Part model, mm, in its own coordinate system. A direction names the side the tool comes from. Give positions to 0.01 mm unless a question says otherwise; leave off trailing zeros.
```python
from build123d import *

# Parameters (mm, degrees)
CROQUIS1_R              = 13.5
SALIENTE_EXTRUIR1_DEPTH = 17
CORTAR_EXTRUIR5_START   = -26
CORTAR_EXTRUIR5_DEPTH   = 26
CROQUIS8_R              = 10
SALIENTE_EXTRUIR2_DEPTH = 5
CROQUIS9_R              = 4.5
CORTAR_EXTRUIR6_DEPTH   = 45
CROQUIS10_R             = 6
CORTAR_EXTRUIR8_DEPTH   = 4
CROQUIS12_R             = 15
SALIENTE_EXTRUIR4_DEPTH = 2.5
CORTAR_EXTRUIR9_START   = -25
CROQUIS13_R             = 4.5
CORTAR_EXTRUIR9_DEPTH   = 25
SALIENTE_EXTRUIR5_START = 0.5
CROQUIS14_R             = 10
SALIENTE_EXTRUIR5_DEPTH = 0.5
CORTAR_EXTRUIR10_START  = -2
CROQUIS15_R             = 6
CORTAR_EXTRUIR10_DEPTH  = 2
CORTAR_EXTRUIR12_DEPTH  = 50
REDONDEO1_R             = 0.5


with BuildPart() as part:
    # Croquis1 → Saliente-Extruir1 (new body)
    with BuildSketch(Plane.XY):
        Circle(CROQUIS1_R)
    extrude(amount=SALIENTE_EXTRUIR1_DEPTH)

    # Croquis2 → Cortar-Extruir5 (cut)
    with BuildSketch(Plane.XY.offset(17).offset(CORTAR_EXTRUIR5_START)):
        with BuildLine():
            ThreePointArc((-6.44082437, 11.864475607), (-3.933231648, 10.806465139), (-2.692380198, 13.228797711))
            ThreePointArc((-2.692380198, 13.228797711), (-4.617271935, 12.685850381), (-6.44082437, 11.864475607))
        make_face()
        with BuildLine():
            ThreePointArc((-10.11028478, 8.946068504), (-7.392057511, 8.809511096), (-7.054525094, 11.510155329))
            ThreePointArc((-7.054525094, 11.510155329), (-8.677632731, 10.341599982), (-10.11028478, 8.946068504))
        make_face()
        with BuildLine():
            ThreePointArc((-12.560295633, 4.948633509), (-9.959292144, 5.75), (-10.565790149, 8.403218343))
            ThreePointArc((-10.565790149, 8.403218343), (-11.691342951, 6.75), (-12.560295633, 4.948633509))
        make_face()
        with BuildLine():
            ThreePointArc((1.994505484, 13.351851852), (0, 13.5), (-1.994505484, 13.351851852))
            ThreePointArc((-1.994505484, 13.351851852), (0, 11.5), (1.994505484, 13.351851852))
        make_face()
        with BuildLine():
            ThreePointArc((6.44082437, 11.864475607), (4.617271935, 12.685850381), (2.692380198, 13.228797711))
            ThreePointArc((2.692380198, 13.228797711), (3.933231648, 10.806465139), (6.44082437, 11.864475607))
        make_face()
        with BuildLine():
            ThreePointArc((10.11028478, 8.946068504), (8.677632731, 10.341599982), (7.054525094, 11.510155329))
            ThreePointArc((7.054525094, 11.510155329), (7.392057511, 8.809511096), (10.11028478, 8.946068504))
        make_face()
        with BuildLine():
            ThreePointArc((12.560295633, 4.948633509), (11.691342951, 6.75), (10.565790149, 8.403218343))
            ThreePointArc((10.565790149, 8.403218343), (9.959292144, 5.75), (12.560295633, 4.948633509))
        make_face()
        with BuildLine():
            ThreePointArc((13.495349463, 0.354320278), (13.294904666, 2.344250399), (12.802664978, 4.282729207))
            ThreePointArc((12.802664978, 4.282729207), (11.32528916, 1.996954043), (13.495349463, 0.354320278))
        make_face()
        with BuildLine():
            ThreePointArc((12.802664978, -4.282729207), (13.294904666, -2.344250399), (13.495349463, -0.354320278))
            ThreePointArc((13.495349463, -0.354320278), (11.32528916, -1.996954043), (12.802664978, -4.282729207))
        make_face()
        with BuildLine():
            ThreePointArc((10.565790149, -8.403218343), (11.691342951, -6.75), (12.560295633, -4.948633509))
            ThreePointArc((12.560295633, -4.948633509), (9.959292144, -5.75), (10.565790149, -8.403218343))
        make_face()
        with BuildLine():
            ThreePointArc((7.054525094, -11.510155329), (8.677632731, -10.341599982), (10.11028478, -8.946068504))
            ThreePointArc((10.11028478, -8.946068504), (7.392057511, -8.809511096), (7.054525094, -11.510155329))
        make_face()
        with BuildLine():
            ThreePointArc((2.692380198, -13.228797711), (4.617271935, -12.685850381), (6.44082437, -11.864475607))
            ThreePointArc((6.44082437, -11.864475607), (3.933231648, -10.806465139), (2.692380198, -13.228797711))
        make_face()
        with BuildLine():
            ThreePointArc((1.994505484, -13.351851852), (0, -11.5), (-1.994505484, -13.351851852))
            ThreePointArc((-1.994505484, -13.351851852), (0, -13.5), (1.994505484, -13.351851852))
        make_face()
        with BuildLine():
            ThreePointArc((-2.692380198, -13.228797711), (-3.933231648, -10.806465139), (-6.44082437, -11.864475607))
            ThreePointArc((-6.44082437, -11.864475607), (-4.617271935, -12.685850381), (-2.692380198, -13.228797711))
        make_face()
        with BuildLine():
            ThreePointArc((-7.054525094, -11.510155329), (-7.392057511, -8.809511096), (-10.11028478, -8.946068504))
            ThreePointArc((-10.11028478, -8.946068504), (-8.677632731, -10.341599982), (-7.054525094, -11.510155329))
        make_face()
        with BuildLine():
            ThreePointArc((-10.565790149, -8.403218343), (-9.959292144, -5.75), (-12.560295633, -4.948633509))
            ThreePointArc((-12.560295633, -4.948633509), (-11.691342951, -6.75), (-10.565790149, -8.403218343))
        make_face()
        with BuildLine():
            ThreePointArc((-12.802664978, -4.282729207), (-11.32528916, -1.996954043), (-13.495349463, -0.354320278))
            ThreePointArc((-13.495349463, -0.354320278), (-13.294904666, -2.344250399), (-12.802664978, -4.282729207))
        make_face()
        with BuildLine():
            ThreePointArc((-13.495349463, 0.354320278), (-11.32528916, 1.996954043), (-12.802664978, 4.282729207))
            ThreePointArc((-12.802664978, 4.282729207), (-13.294904666, 2.344250399), (-13.495349463, 0.354320278))
        make_face()
    extrude(amount=CORTAR_EXTRUIR5_DEPTH, mode=Mode.SUBTRACT)

    # Croquis8 → Saliente-Extruir2 (add)
    with BuildSketch(Plane.XY.offset(17)):
        Circle(CROQUIS8_R)
    extrude(amount=SALIENTE_EXTRUIR2_DEPTH)

    # Croquis9 → Cortar-Extruir6 (cut)
    with BuildSketch(Plane.XY.offset(22)):
        Circle(CROQUIS9_R)
    extrude(amount=-CORTAR_EXTRUIR6_DEPTH, mode=Mode.SUBTRACT)

    # Croquis10 → Cortar-Extruir8 (cut)
    with BuildSketch(Plane.XY.offset(22)):
        Circle(CROQUIS10_R)
    extrude(amount=-CORTAR_EXTRUIR8_DEPTH, mode=Mode.SUBTRACT)

    # Croquis12 → Saliente-Extruir4 (add)
    with BuildSketch(Plane(origin=(0, 0, 0), x_dir=(-1, 0, 0), z_dir=(0, 0, -1))):
        Circle(CROQUIS12_R)
    extrude(amount=SALIENTE_EXTRUIR4_DEPTH)

    # Croquis13 → Cortar-Extruir9 (cut)
    with BuildSketch(Plane(origin=(0, 0, -2.5), x_dir=(-1, 0, 0), z_dir=(0, 0, -1)).offset(CORTAR_EXTRUIR9_START)):
        with Locations(Location((0, 0, 0), (0, 0, 180))):
            Circle(CROQUIS13_R)
    extrude(amount=CORTAR_EXTRUIR9_DEPTH, mode=Mode.SUBTRACT)

    # Croquis14 → Saliente-Extruir5 (add)
    with BuildSketch(Plane(origin=(0, 0, -2.5), x_dir=(-1, 0, 0), z_dir=(0, 0, -1)).offset(SALIENTE_EXTRUIR5_START)):
        with Locations(Location((0, 0, 0), (0, 0, 180))):
            Circle(CROQUIS14_R)
    extrude(amount=-SALIENTE_EXTRUIR5_DEPTH)

    # Croquis15 → Cortar-Extruir10 (cut)
    with BuildSketch(Plane(origin=(0, 0, -3), x_dir=(-1, 0, 0), z_dir=(0, 0, -1)).offset(CORTAR_EXTRUIR10_START)):
        with Locations(Location((0, 0, 0), (0, 0, 180))):
            Circle(CROQUIS15_R)
    extrude(amount=CORTAR_EXTRUIR10_DEPTH, mode=Mode.SUBTRACT)

    # Croquis16 → Cortar-Extruir12 (cut)
    with BuildSketch(Plane.XY.offset(22)):
        with BuildLine():
            Line((-1.5, 4.242640687), (-1.5, 5.812640687))
            Line((-1.5, 5.812640687), (1.5, 5.812640687))
            Line((1.5, 5.812640687), (1.5, 4.242640687))
            ThreePointArc((1.5, 4.242640687), (0, 4.5), (-1.5, 4.242640687))
        make_face()
    extrude(amount=-CORTAR_EXTRUIR12_DEPTH, mode=Mode.SUBTRACT)

    # Redondeo1
    redondeo1_edges = [part.edges().sort_by_distance(p)[0] for p in [
        (15, 0, 0),
    ]]
    fillet(redondeo1_edges, radius=REDONDEO1_R)


solid = part.part
```
1) Wall check: L1, parallel to X at y = -11.25, z = 5.75; L2, parallel to Y at x = 0, z = 19.1; L3, parallel to X at y = 0, z = 3. Give the ranges that are in metal, low to high.
Answers follow:
L1: x = -6.9 to -6.01, -3.23 to 3.23, 6.01 to 6.9
L2: y = -10 to -6, 6 to 10
L3: x = -13.5 to -4.5, 4.5 to 13.5
2) 3-axis set-ups, long thin cutter, end or side, ignore diameter. For faces 5 (the face through (2.2, -4.1, -1)), 6 (the face through (0, -6, 20)), 7 (the face through (0, 7, -3)), 8 (the face through (1.5, 5, 10)), 9 (the face through (0, 11.5, 8.4)): which of +Z, -Z, +X, -X, +Y, -Y reach the whole face in a straight line?
Answers follow:
face 5: -Z
face 6: +Z
face 7: -Z, +X, -X, +Y, -Y
face 8: +Z, -Z
face 9: +Z, +Y
3) Pin check, flat tips, straight feed: pin 1 Ø4 at (y, z) = (-5.5, 15.5) entering from -X; pin 2 Ø5 at (x, z) = (2, 16) entering from -Y; pin 3 Ø1.5 at (y, z) = (12, 1.5) entering from -X; pin 4 Ø9.5 at (x, y) = (3, -1.5) entering from +Z. Stop position of each tip, or through.
Answers follow:
pin 1: stops at x = -12.8
pin 2: stops at y = -13.35
pin 3: stops at x = -7.05
pin 4: stops at z = 22
4) Two-plate mould, pull along Y, no slides. Class faces 1 (the face through (-11.333, 1.956, 8.381)), 2 (the face through (14.985, 0.66, -1.486)), 3 (the face through (0, -11.5, 8.4)), 4 (the face through (0, 6, 20)): +Y half, -Y half, draft (parallel to the pull), parting line (faces both ways), or undercut.
Answers follow:
face 1: undercut
face 2: parting line
face 3: -Y half
face 4: undercut
